For this review, use the dimensioned drawing (mm, ordinates from the lowest corner) and the shaded views. A direction names the side the tool comes from. Round coordinates to 2 decimals unless told otherwise and drop trailing zeros. Order: outer loops, then holes, each group sorted by start corner. A loop starts at its lowest first (then second) coordinate and runs counter-clockwise, first axis right, second up. Notation, with made-up numbers: M -28,64 L 19,64 A11 cw 19,80 Z; hole C 11,83.5 d10. An arc over 180 degrees is marked long. Put each result on its own line as item: value.
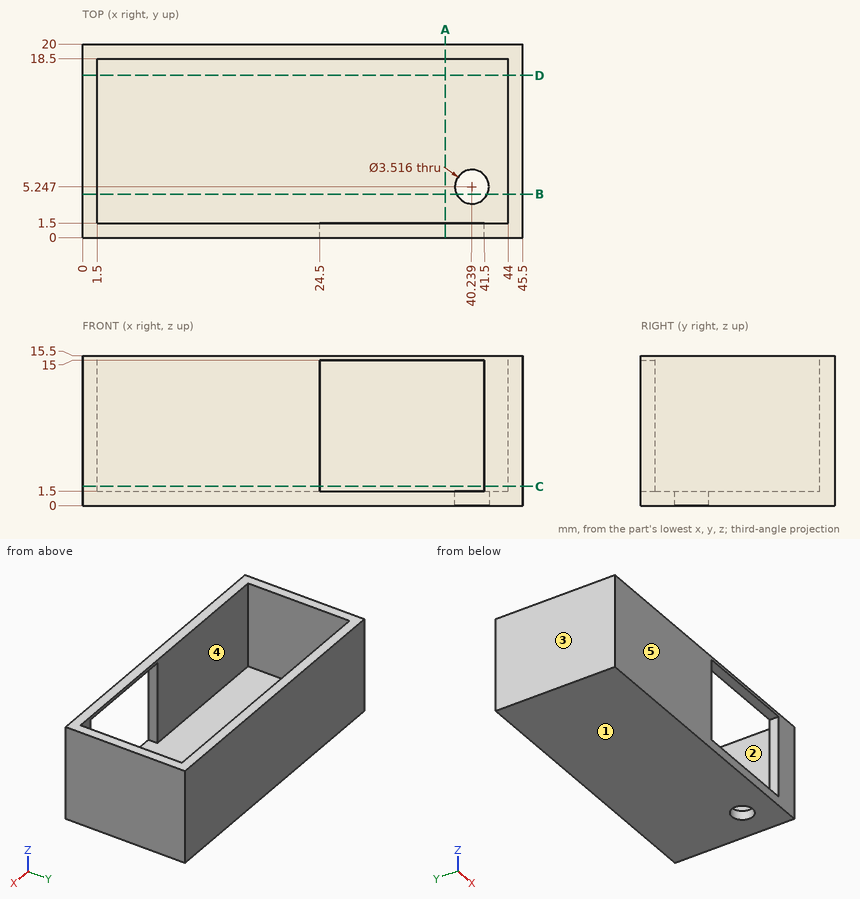
(1) To check wall thickness, follow L1, parallel to X at y = 10.25, z = 11.75; L2, parallel to Y at x = 19, z = 4; L3, parallel to Z at x = 3, y = 13. State the ranges of each line that lie inside material, in increasing order.
A:
L1: x = 0 to 1.5, 44 to 45.5
L2: y = 0 to 1.5, 18.5 to 20
L3: z = 0 to 1.5
(2) Draft analysis for pull direction Y (two halves, no side actions). For the marked faces 3, 4 and 5, state which applies: released by +Y, released by -Y, zero draft, split by the parting line, or undercut.
A:
face 3: zero draft
face 4: undercut
face 5: released by -Y
(3) For the marked faces 1 and 2, list the 3-axis set-ups (+Z, -Z, +X, -X, +Y, -Y) from which the entire face can be reached by the end or side of a thin tool; tool diameter is ignored.
A:
face 1: -Z, +X, -X, +Y, -Y
face 2: +Z
(4) Add section B-B on y = 4.5. Give the boundary of the cut face in (x, z).
A:
outline: M 0,0 L 38.65,0 L 38.65,1.5 L 1.5,1.5 L 1.5,15.5 L 0,15.5 Z; M 41.83,0 L 45.5,0 L 45.5,15.5 L 44,15.5 L 44,1.5 L 41.83,1.5 Z
(5) Add section D-D on y = 16.75. Give the boundary of the cut face in (x, z), then the cut area to 3 significant figures.
A:
outline: M 0,0 L 45.5,0 L 45.5,15.5 L 44,15.5 L 44,1.5 L 1.5,1.5 L 1.5,15.5 L 0,15.5 Z
area: 110 mm2
(6) Add section A-A on x = 37.5. Give the boundary of the cut face in (y, z).
A:
outline: M 0,0 L 20,0 L 20,15.5 L 18.5,15.5 L 18.5,1.5 L 0,1.5 Z; M 0,15 L 1.5,15 L 1.5,15.5 L 0,15.5 Z
(7) Add section C-C on z = 2. Give the boundary of the cut face in (x, y).
A:
outline: M 0,0 L 24.5,0 L 24.5,1.5 L 1.5,1.5 L 1.5,18.5 L 44,18.5 L 44,1.5 L 41.5,1.5 L 41.5,0 L 45.5,0 L 45.5,20 L 0,20 Z
(8) Insertion check: pin 1 Ø1.5 at (x, z) = (27, 7.5) entering from -Y; pin 2 Ø1.5 at (x, y) = (8.5, 16.5) entering from +Z; pin 3 Ø7 at (x, z) = (22, 10.5) entering from -Y. Each pin has a flat end and moves straight along its axis. Give the tip position at first contact, or say it passes through.
A:
pin 1: stops at y = 18.5
pin 2: stops at z = 1.5
pin 3: stops at y = 0
